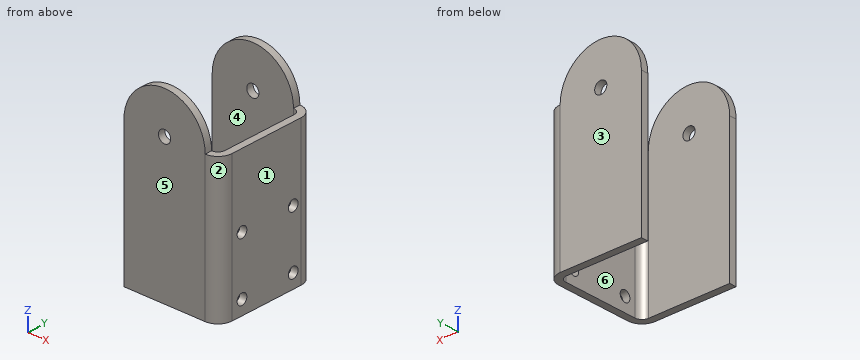
```python
from build123d import *

# Parameters (mm, degrees)
BASE_FLANGE1_DEPTH      = 63.5
BOSS_EXTRUDE1_DEPTH     = 3.175
BOSS_EXTRUDE2_START     = -3.175
BOSS_EXTRUDE2_DEPTH     = 3.175
SKETCH8_R               = 2.413
CUT_EXTRUDE1_DEPTH      = 3.175
CUT_EXTRUDE2_DEPTH      = 103.459665412
CUT_EXTRUDE2_DEPTH_BACK = 103.459665412
SKETCH10_R              = 2.753999953


# Sheet-metal steps are written as plain solids
with BuildPart() as part:
    # Sketch1 → Base-Flange1 (new body)
    with BuildSketch(Plane.XY):
        with BuildLine():
            Line((-39.878, -20.32), (-3.175, -20.32))
            ThreePointArc((-3.175, -20.32), (-0.92993597, -19.39006403), (0, -17.145))
            Line((0, -17.145), (0, 17.145))
            ThreePointArc((0, 17.145), (-0.92993597, 19.39006403), (-3.175, 20.32))
            Line((-3.175, 20.32), (-39.878, 20.32))
            Line((-39.878, 20.32), (-39.878, 23.495))
            Line((-39.878, 23.495), (-3.175, 23.495))
            ThreePointArc((-3.175, 23.495), (1.315128061, 21.635128061), (3.175, 17.145))
            Line((3.175, 17.145), (3.175, -17.145))
            ThreePointArc((3.175, -17.145), (1.315128061, -21.635128061), (-3.175, -23.495))
            Line((-3.175, -23.495), (-39.878, -23.495))
            Line((-39.878, -23.495), (-39.878, -20.32))
        make_face()
    extrude(amount=BASE_FLANGE1_DEPTH)

    # Sketch6 → Boss-Extrude1 (add)
    with BuildSketch(Plane(origin=(0, 23.495, 0), x_dir=(1, 0, 0), z_dir=(0, 1, 0))):
        with BuildLine():
            Line((-39.878, -63.5), (-3.175, -63.5))
            ThreePointArc((-3.175, -63.5), (-21.5265, -81.8515), (-39.878, -63.5))
        make_face()
    extrude(amount=-BOSS_EXTRUDE1_DEPTH)

    # Sketch7 → Boss-Extrude2 (add)
    with BuildSketch(Plane.XZ.offset(23.495).offset(BOSS_EXTRUDE2_START)):
        with BuildLine():
            Line((-3.175, 63.5), (-39.878, 63.5))
            ThreePointArc((-39.878, 63.5), (-21.5265, 81.8515), (-3.175, 63.5))
        make_face()
    extrude(amount=BOSS_EXTRUDE2_DEPTH)

    # Sketch8 → Cut-Extrude1 (cut)
    with BuildSketch(Plane(origin=(3.175, 0, 0), x_dir=(0, 0, -1), z_dir=(1, 0, 0))):
        with Locations(Location((-6.35, 13.18662794, 0), (0, 0, 90))):
            Circle(SKETCH8_R)
        with Locations(Location((-31.75, 13.18662794, 0), (0, 0, 90))):
            Circle(SKETCH8_R)
        with Locations(Location((-31.75, -12.21337206, 0), (0, 0, 90))):
            Circle(SKETCH8_R)
        with Locations(Location((-6.35, -12.21337206, 0), (0, 0, 90))):
            Circle(SKETCH8_R)
    extrude(amount=-CUT_EXTRUDE1_DEPTH, mode=Mode.SUBTRACT)

    # Sketch10 → Cut-Extrude2 (cut, two sides: drawn at the far end of the back side and taken through both)
    with BuildSketch(Plane(origin=(0, 23.495, 0), x_dir=(1, 0, 0), z_dir=(0, 1, 0)).offset(-CUT_EXTRUDE2_DEPTH_BACK)):
        with Locations(Location((-21.5265, -63.5, 0), (0, 0, 180))):
            Circle(SKETCH10_R)
    extrude(amount=CUT_EXTRUDE2_DEPTH + CUT_EXTRUDE2_DEPTH_BACK, mode=Mode.SUBTRACT)


solid = part.part
```
Geometry check sheet. Reference: the model listing, model coordinates, mm. Face numbers are marked on the shaded views. A direction names the side the tool comes from. Give positions to 0.01 mm unless a question says otherwise; leave off trailing zeros. Order: outer loops, then holes, each group sorted by start corner. A loop starts at its lowest first (then second) coordinate and runs counter-clockwise, first axis right, second up. Notation, with made-up numbers: (11, 1) - (48, 1) arc R16 cw to (48, 31) - close; hole circle Ø4 at (61, 74). An arc over 180 degrees is marked (long way). Answer in a Markdown table with one row per item. Add a question column.
Q1. Material ranges on probe 1 along Y at (x, z) = (-28.5, 31) (3 decimals); probe 2 along Z at (x, y) = (-0.5, -19); probe 3 along X at (y, z) = (-7, 15) (3 decimals), recorded low to high. Write a range as from..to.
Q2. Mould release check, pull along Y, two halves, no side actions. Record for the marked faces 1, 2, 3 and 4: pulls with the +Y half, pulls with the -Y half, needs draft (parallel to the pull), parting line crosses it, or undercut.
Q3. Gauge pin test, flat ends, axial feed: pin 1 (10 mm diameter, centred on y = 15.5, z = 68.5, fed in from -X); pin 2 (7.5 mm diameter, centred on y = -12.21, z = 6.35, fed in from -X). Record the tip position at first contact, or that the pin passes through.
Q4. Cross-section at B-B, the plane x = -22.5. Enter the section's corners in (y, z) (3 decimals).
Q5. Cross-section at C-C, the plane x = -7. Enter the section's corners in (y, z) (3 decimals), then the cut area to 3 significant figures.
Q6. Cross-section at A-A, the plane z = 6.35. Enter the section's corners in (x, y) (3 decimals), then the cut area to 3 significant figures.
Q7. Tool access check on the marked faces 5 and 6. Record the directions out of +Z, -Z, +X, -X, +Y, -Y that give a thin tool (end or side, any length) a straight path to the whole face; none if there is none.
Q8. Cross-section at D-D, the plane z = 43. Enter the section's corners in (x, y) (3 decimals), then the cut area to 3 significant figures.
Check values:
| question | item | result |
|---|---|---|
| 1 | probe 1 | y = -23.495..-20.32, 20.32..23.495 |
| 1 | probe 2 | z = 0..63.5 |
| 1 | probe 3 | x = 0..3.175 |
| 2 | face 1 | needs draft |
| 2 | face 2 | pulls with the -Y half |
| 2 | face 3 | pulls with the +Y half |
| 2 | face 4 | undercut |
| 3 | pin 1 | stops at x = -39.51 |
| 3 | pin 2 | stops at x = 0 |
| 4 | outline | (-23.495, 0) - (-20.32, 0) - (-20.32, 60.924) - (-23.495, 60.924) - close; (-23.495, 66.076) - (-20.32, 66.076) - (-20.32, 81.826) - (-23.495, 81.826) - close; (20.32, 0) - (23.495, 0) - (23.495, 60.924) - (20.32, 60.924) - close; (20.32, 66.076) - (23.495, 66.076) - (23.495, 81.826) - (20.32, 81.826) - close |
| 5 | outline | (-23.495, 0) - (-20.32, 0) - (-20.32, 74.714) - (-23.495, 74.714) - close; (20.32, 0) - (23.495, 0) - (23.495, 74.714) - (20.32, 74.714) - close |
| 5 | area | 474 mm^2 |
| 6 | outline | (-39.878, -23.495) - (-3.175, -23.495) arc R6.35 ccw to (3.175, -17.145) - (3.175, -14.626) - (0, -14.626) - (0, -17.145) arc R3.175 cw to (-3.175, -20.32) - (-39.878, -20.32) - close; (-39.878, 20.32) - (-3.175, 20.32) arc R3.175 cw to (0, 17.145) - (0, 15.6) - (3.175, 15.6) - (3.175, 17.145) arc R6.35 ccw to (-3.175, 23.495) - (-39.878, 23.495) - close; (0, -9.8) - (3.175, -9.8) - (3.175, 10.774) - (0, 10.774) - close |
| 6 | area | 359 mm^2 |
| 7 | face 5 | +Z, -Z, +X, -X, -Y |
| 7 | face 6 | +Z, -Z, -X |
| 8 | outline | (-39.878, -23.495) - (-3.175, -23.495) arc R6.35 ccw to (3.175, -17.145) - (3.175, 17.145) arc R6.35 ccw to (-3.175, 23.495) - (-39.878, 23.495) - (-39.878, 20.32) - (-3.175, 20.32) arc R3.175 cw to (0, 17.145) - (0, -17.145) arc R3.175 cw to (-3.175, -20.32) - (-39.878, -20.32) - close |
| 8 | area | 389 mm^2 |
